Here's the drawing with two shaded views (mm, measured from the low corner). I have some questions. A direction names the side the tool comes from. Coordinates: 2 decimals unless noted, no trailing zeros. Write each loop counter-clockwise with the first axis right and the second up, starting at its lowest first coordinate (ties: lowest second). Pieces come first, ordered by that corner, then holes.
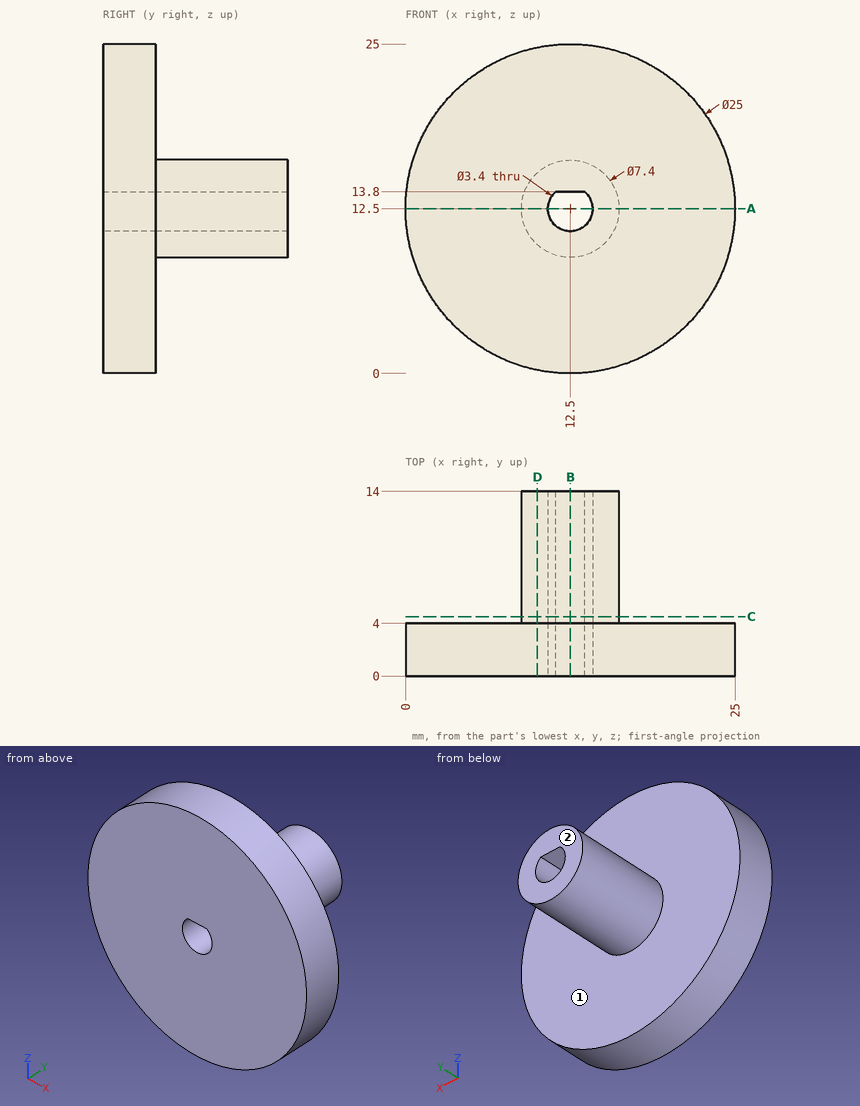
1. I want a section at A-A on z = 12.5. Please give me the cut outline in (x, y), plus the area to 3 significant figures.
Verdict:
outline: (0, 0) - (10.8, 0) - (10.8, 14) - (8.8, 14) - (8.8, 4) - (0, 4) - close; (14.2, 0) - (25, 0) - (25, 4) - (16.2, 4) - (16.2, 14) - (14.2, 14) - close
area: 126 mm2
2. Please list where these lines run through material, in increasing order: line 1 along X through (y, z) = (9.5, 12.5); line 2 along X through (y, z) = (3.05, 12.5); line 3 along Z through (x, y) = (12.5, 2.55).
Verdict:
line 1: x = 8.8 to 10.8, 14.2 to 16.2
line 2: x = 0 to 10.8, 14.2 to 25
line 3: z = 0 to 10.8, 13.8 to 25
3. I want a section at C-C on y = 4.5. Please give me the cut outline in (x, z), plus the area to 3 significant figures.
Verdict:
outline: circle Ø7.4 at (12.5, 12.5); hole (11.4, 13.8) arc R1.7 ccw (long way) to (13.6, 13.8) - close
area: 34.5 mm2
4. I want a section at B-B on x = 12.5. Please give me the cut outline in (y, z).
Verdict:
outline: (0, 0) - (4, 0) - (4, 8.8) - (14, 8.8) - (14, 10.8) - (0, 10.8) - close; (0, 13.8) - (14, 13.8) - (14, 16.2) - (4, 16.2) - (4, 25) - (0, 25) - close
5. I want a section at D-D on x = 10. Please give me the cut outline in (y, z).
Verdict:
outline: (0, 0.25) - (4, 0.25) - (4, 9.77) - (14, 9.77) - (14, 15.23) - (4, 15.23) - (4, 24.75) - (0, 24.75) - close
6. On a 3-axis mill with a long thin cutter (end or side, diameter ignored), from which of +Z, -Z, +X, -X, +Y, -Y can I reach the whole of each face in a straight line? I mean the marked faces 1 and 2. Say none if no direction works.
Verdict:
face 1: +Y
face 2: +Z, -Z, +X, -X, +Y
7. For pin 1 (2.5 mm diameter, centred on x = 12.5, z = 12.5, fed in from +Y); pin 2 (6 mm diameter, centred on x = 9, z = 3.5, fed in from +Y); pin 3 (1 mm diameter, centred on x = 10, y = 11.5, fed in from -Z); pin 4 (8 mm diameter, centred on x = 8, y = 4.5, fed in from -Z), each with a flat end and sliding along its axis, tell me the tip position at first contact or that it passes through.
Verdict:
pin 1: passes through
pin 2: stops at y = 4
pin 3: stops at z = 9.39
pin 4: stops at z = 0.01
